The model under review builds one solid part; all positions refer to its coordinate system, in mm. Face numbers are marked on the shaded views. A direction names the side the tool comes from. Round coordinates to 2 decimals unless told otherwise and drop trailing zeros. Write each loop counter-clockwise with the first axis right and the second up, starting at its lowest first coordinate (ties: lowest second). Pieces come first, ordered by that corner, then holes. Notation, with made-up numbers: (64.25, 10.25) -> (75.25, 10.25) arc R22 cw to (75.25, 44.25) -> close; hole circle Ø4 at (71, 69.5). An arc over 180 degrees is marked (long way). Answer as a JSON object with one key per item and string values. Group by question number.
1) We need section B-B, the plane z = 1.9. Write out the cut boundary in (x, y), then the cut area to 3 significant figures.
2) We need section A-A, the plane z = 0.5. Write out the cut boundary in (x, y).
3) Machinability: for the marked faces 3 and 4, which of the approach directions +Z, -Z, +X, -X, +Y, -Y give a long, thin tool a straight path to every point of the face, cutting with its end or side? Answer none if there is none.
4) To check wall thickness, follow probe 1 along X at (y, z) = (0.5, 1.4); probe 2 along Z at (x, y) = (-2.25, 6); probe 3 along X at (y, z) = (1.75, 1.95). State the ranges of each line that lie inside material, in increasing order. Write a range as [from, to].
5) Insertion check: pin 1 Ø4.5 at (x, y) = (2, -1.5) entering from +Z; pin 2 Ø1 at (x, z) = (-6, 1) entering from -Y. Each pin has a flat end and moves straight along its axis. Give the tip position at first contact, or say it passes through.
6) Mouldability with a two-part tool opening along X and no side actions: class the marked faces 1 and 2 as pulls with the +X half, pulls with the -X half, needs draft (parallel to the pull), parting line crosses it, or undercut.
from build123d import *

# Parameters (mm, degrees)
F1_DEPTH = 2.5
F0_R     = 1.25
F2_DEPTH = 1.5
F3_R     = 1


with BuildPart() as f1:
    # F0 (on Top) → F1 (new body)
    with BuildSketch(Plane.XY):
        with BuildLine():
            ThreePointArc((0, 7.5), (5.3033008589, 5.3033008589), (7.5, 0))
            ThreePointArc((7.5, 0), (5.3033008589, -5.3033008589), (0, -7.5))
            Line((0, -7.5), (0, -10))
            ThreePointArc((0, -10), (7.0710678119, -7.0710678119), (10, 0))
            ThreePointArc((10, 0), (7.0710678119, 7.0710678119), (0, 10))
            Line((0, 10), (0, 7.5))
        make_face()
        with BuildLine():
            ThreePointArc((0, -7.5), (-7.5, 0), (0, 7.5))
            Line((0, 7.5), (0, 10))
            ThreePointArc((0, 10), (-10, 0), (0, -10))
            Line((0, -10), (0, -7.5))
        make_face()
    extrude(amount=F1_DEPTH)

    # F0 (on Top) → F2 (join)
    with BuildSketch(Plane.XY):
        with BuildLine():
            Line((0, -7.5), (0, 7.5))
            ThreePointArc((0, 7.5), (-7.5, 0), (0, -7.5))
        make_face()
        with Locations((-3.3498867415, 0)):
            Circle(F0_R, mode=Mode.SUBTRACT)
        with BuildLine():
            ThreePointArc((0, -7.5), (5.3033008589, -5.3033008589), (7.5, 0))
            ThreePointArc((7.5, 0), (5.3033008589, 5.3033008589), (0, 7.5))
            Line((0, 7.5), (0, -7.5))
        make_face()
        with Locations((3.3498867415, 0)):
            Circle(F0_R, mode=Mode.SUBTRACT)
    extrude(amount=F2_DEPTH)

    # F3
    f3_edges = [f1.edges().sort_by_distance(p)[0] for p in [
        (-10, 0, 2.5),
    ]]
    fillet(f3_edges, radius=F3_R)


solid = f1.part
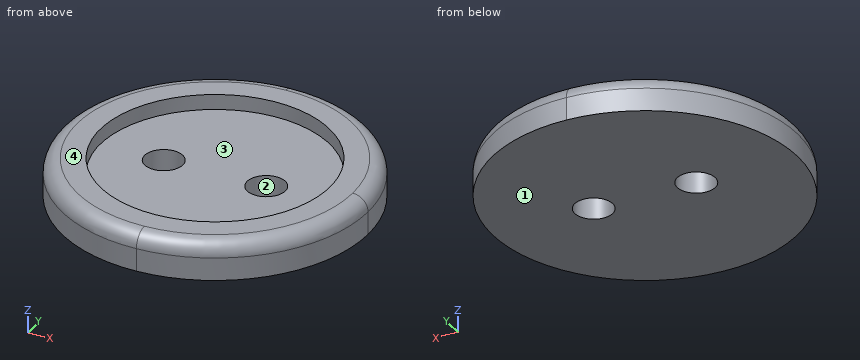
Here are the results:
{
 "1": {"outline": "circle Ø19.83 at (0, 0); hole circle Ø15 at (0, 0)", "area": "132 mm^2"},
 "2": {"outline": "circle Ø20 at (0, 0); hole circle Ø2.5 at (-3.35, 0); hole circle Ø2.5 at (3.35, 0)"},
 "3": {"face 3": "+Z", "face 4": "+Z, +X, -X, +Y, -Y"},
 "4": {"probe 1": "x = [-9.99, -4.5], [-2.2, 2.2], [4.5, 9.99]", "probe 2": "z = [0, 1.5]", "probe 3": "x = [-9.74, -7.29], [7.29, 9.74]"},
 "5": {"pin 1": "stops at z = 1.5", "pin 2": "stops at y = -8.35"},
 "6": {"face 1": "needs draft", "face 2": "undercut"}
}
